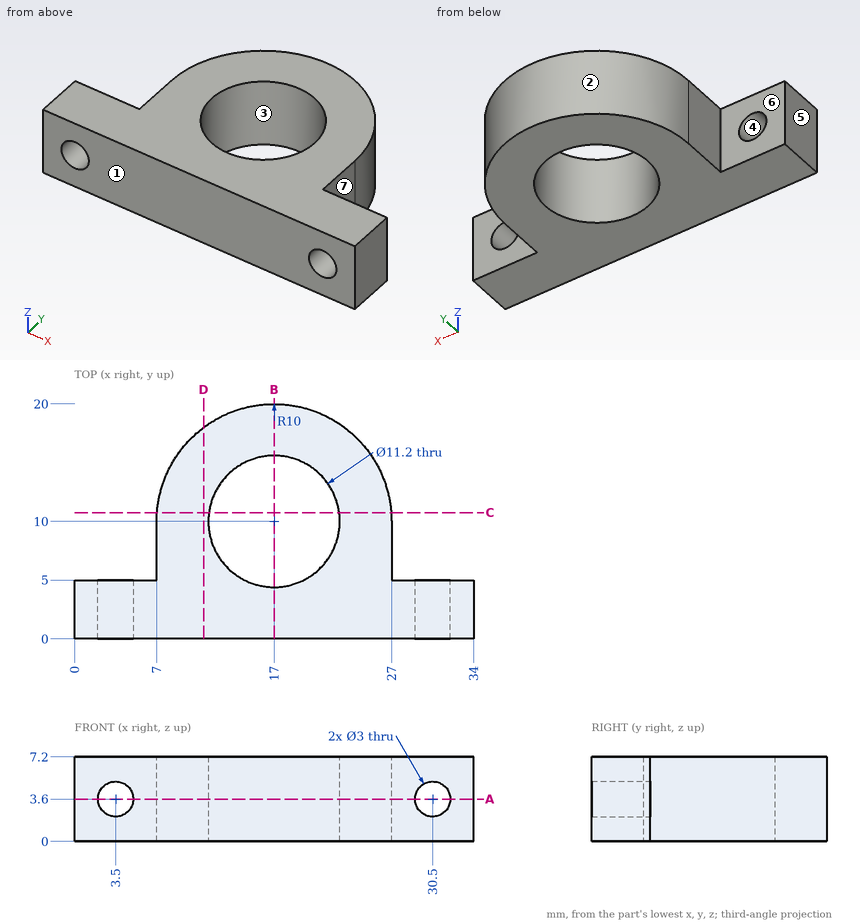
Verification items for this drawing (mm, ordinates from the low corner). A direction names the side the tool comes from. Coordinates: 2 decimals unless noted, no trailing zeros. Loops run counter-clockwise (first coordinate to the right, second up) from the corner with the lowest first, then second, coordinate; pieces in that order, holes last. Notation, with made-up numbers: (30.25, 31.5) -> (69.25, 31.5) arc R21 ccw to (69.25, 48.5) -> close; hole circle Ø5 at (69, 62). An arc over 180 degrees is marked (long way). Put each result on its own line as item: value.
1. Gauge pin test, flat ends, axial feed: P1, Ø2.5, axis at y = 7.5, z = 4.5, coming from the -X side; P2, Ø4, axis at y = 8, z = 5, coming from the +X side; P3, Ø5, axis at x = 7.5, y = 6.5, coming from the -Z side. Record the tip position at first contact, or that the pin passes through.
Result set:
P1: stops at x = 7
P2: stops at x = 27
P3: stops at z = 0
2. Thickness scan on line 1 (Y direction, x = 17, z = 2.75); line 2 (Z direction, x = 3.5, y = 3.9); line 3 (X direction, y = 9.75, z = 2.25). Record the ranges inside material, lowest first.
Result set:
line 1: y = 0 to 4.4, 15.6 to 20
line 2: z = 0 to 2.1, 5.1 to 7.2
line 3: x = 7 to 11.41, 22.59 to 27
3. Section check B-B, the plane x = 17. Record the boundary of the cut face in (y, z), then the cut area to 3 significant figures.
Result set:
outline: (0, 0) -> (4.4, 0) -> (4.4, 7.2) -> (0, 7.2) -> close; (15.6, 0) -> (20, 0) -> (20, 7.2) -> (15.6, 7.2) -> close
area: 63.4 mm^2
4. Section check D-D, the plane x = 11. Record the boundary of the cut face in (y, z), then the cut area to 3 significant figures.
Result set:
outline: (0, 0) -> (18, 0) -> (18, 7.2) -> (0, 7.2) -> close
area: 130 mm^2
5. Tool access check on the marked faces 5, 6 and 7. Record the directions out of +Z, -Z, +X, -X, +Y, -Y that give a thin tool (end or side, any length) a straight path to the whole face; none if there is none.
Result set:
face 5: +Z, -Z, -X, +Y, -Y
face 6: +Z, -Z, -X, +Y
face 7: +Z, -Z, +X, +Y
6. Section check A-A, the plane z = 3.6. Record the boundary of the cut face in (x, y).
Result set:
outline: (0, 0) -> (2, 0) -> (2, 5) -> (0, 5) -> close; (5, 0) -> (29, 0) -> (29, 5) -> (27, 5) -> (27, 10) arc R10 ccw to (7, 10) -> (7, 5) -> (5, 5) -> close; (32, 0) -> (34, 0) -> (34, 5) -> (32, 5) -> close; hole circle Ø11.2 at (17, 10)
7. Section check C-C, the plane y = 10.75. Record the boundary of the cut face in (x, z).
Result set:
outline: (7.03, 0) -> (11.45, 0) -> (11.45, 7.2) -> (7.03, 7.2) -> close; (22.55, 0) -> (26.97, 0) -> (26.97, 7.2) -> (22.55, 7.2) -> close
8. Mould release check, pull along Y, two halves, no side actions. Record for the marked faces 1, 2, 3 and 4: pulls with the +Y half, pulls with the -Y half, needs draft (parallel to the pull), parting line crosses it, or undercut.
Result set:
face 1: pulls with the -Y half
face 2: pulls with the +Y half
face 3: undercut
face 4: needs draft
